The model under review builds one solid part; all positions refer to its coordinate system, in mm. A direction names the side the tool comes from. Coordinates: 2 decimals unless noted, no trailing zeros. Order: outer loops, then holes, each group sorted by start corner. A loop starts at its lowest first (then second) coordinate and runs counter-clockwise, first axis right, second up. Notation, with made-up numbers: (54, 50) -> (68, 50) arc R8 ccw to (68, 62) -> close; hole circle Ø11 at (24.25, 30). An arc over 180 degrees is marked (long way). Put each result on its own line as item: value.
Autodesk Inventor part; units mm, degrees
ref_plane "YZ Plane" through (0, 0, 0) normal (1, 0, 0) x (0, 1, 0)
ref_plane "XZ Plane" through (0, 0, 0) normal (0, 1, 0) x (-1, 0, 0)
ref_plane "XY Plane" through (0, 0, 0) normal (0, 0, 1) x (1, 0, 0)
sketch "Sketch1" plane through (0, 0, 0) normal (0, 0, 1) x (1, 0, 0)
  line L0 (-16.2013, 52.9706) -> (47.2987, 52.9706)
  line L1 (47.2987, 52.9706) -> (47.2987, -10.5294)
  line L2 (47.2987, -10.5294) -> (-16.2013, -10.5294)
  line L3 (-16.2013, -10.5294) -> (-16.2013, 52.9706)
  point P0 (0, 0)
  dimension "d0" = 63.5
  dimension "d1" = 63.5
extrude "Extrusion1" add sketch "Sketch1" along normal blind 6.35
sketch "Sketch2" plane through (0, 0, 6.35) normal (0, 0, 1) x (1, 0, 0)
  line L0 (-16.2013, -10.5294) -> (-16.2013, 52.9706)
  line L1 (47.2987, -10.5294) -> (-16.2013, -10.5294)
  point P0 (0, 0)
  point P1 (15.5487, 21.2206)
  dimension "d4" = 31.75
  dimension "d5" = 31.75
hole "Hole1" at (15.5487, 21.2206, 6.35) direction (0, 0, -1) diameter 44.323 end through all
sketch "Sketch3" plane through (0, 0, 6.35) normal (0, 0, 1) x (1, 0, 0)
  line L0 (47.2987, 52.9706) -> (47.2987, -10.5294)
  line L1 (-16.2013, 52.9706) -> (47.2987, 52.9706)
  line L2 (-16.2013, -10.5294) -> (-16.2013, 52.9706)
  line L3 (47.2987, -10.5294) -> (-16.2013, -10.5294)
  point P0 (0, 0)
  point P1 (-3.5013, 46.6206)
  point P2 (34.5987, 46.6206)
  point P3 (-3.5013, -4.1794)
  point P4 (34.5987, -4.1794)
  dimension "d13" = 6.35
  dimension "d14" = 12.7
  dimension "d15" = 12.7
  dimension "d16" = 6.35
  dimension "d24" = 12.7
  dimension "d25" = 12.7
hole "Hole2" at (-3.5013, 46.6206, 6.35) at (34.5987, 46.6206, 6.35) at (-3.5013, -4.1794, 6.35) at (34.5987, -4.1794, 6.35) direction (0, 0, -1) diameter 6.096 end through all
sketch "Sketch4" plane through (0, 0, 6.35) normal (0, 0, 1) x (1, 0, 0)
  line L0 (-16.2013, 52.9706) -> (47.2987, 52.9706)
  line L1 (-4.7209, 20.4332) -> (-21.033, 20.4332)
  line L2 (-21.033, 20.4332) -> (-21.033, 22.0207)
  line L3 (-21.033, 22.0207) -> (-4.7209, 22.0207)
  line L4 (-4.7209, 22.0207) -> (-4.7209, 20.4332)
  point P0 (0, 0)
  dimension "d26" = 1.5875
  dimension "d27" = 30.9499
extrude "Extrusion2" cut sketch "Sketch4" against normal blind 6.35
sketch "Sketch5" plane through (-16.2013, 52.9706, 0) normal (0, 1, 0) x (1, 0, 0)
  line L0 (0, 0) -> (63.5, 0)
  line L1 (0, 0) -> (0, -6.35)
  point P0 (16.2013, 0)
  point P1 (3.175, -3.175)
  dimension "d30" = 3.175
  dimension "d31" = 3.175
hole "Hole3" at (-13.0263, 52.9706, 3.175) direction (0, -1, 0) diameter 2.6416 depth 50.8 tip angle 118
sketch "Sketch6" plane through (-16.2013, 52.9706, 0) normal (0, 1, 0) x (1, 0, 0)
  circle A0 centre (3.175, -3.175) radius 1.3208
  point P0 (16.2013, 0)
hole "Hole4" at (-13.0263, 52.9706, 3.175) direction (0, -1, 0) diameter 3.81 depth 31.75 tip angle 118
sketch "Sketch7" plane through (0, 0, 0) normal (0, 0, -1) x (-1, 0, 0)
  line L0 (-47.2987, 52.9706) -> (-47.2987, -10.5294)
  line L1 (-40.9487, 22.0207) -> (-35.1672, 22.0207)
  line L2 (-35.1672, 22.0207) -> (-35.1672, 20.4332)
  line L3 (-35.1672, 20.4332) -> (-40.9487, 20.4332)
  line L4 (-40.9487, 20.4332) -> (-40.9487, 22.0207)
  point P0 (0, 0)
  dimension "d46" = 6.35
extrude "Extrusion3" cut sketch "Sketch7" against normal blind 6.35
properties part number "JF-AT-JC0015" material "Aluminum-6061 (Anodized Black)"
Item 1: Consider section D-D on y = 8. Write out the cut boundary in (x, z) (3 decimals), and give its area (3 significant figures).
Answers below:
outline: (-16.201, 0) -> (-2.237, 0) -> (-2.237, 6.35) -> (-16.201, 6.35) -> close; (33.335, 0) -> (47.299, 0) -> (47.299, 6.35) -> (33.335, 6.35) -> close; hole circle Ø2.642 at (-13.026, 3.175)
area: 172 mm^2
Item 2: For faces 1 (the cylindrical face through (-14.336, 11.174, 3.003)), 2 (the flat face through (39, 22.021, 3)), 3 (the flat face through (47.299, 22, 3)), list the 3-axis set-ups (+Z, -Z, +X, -X, +Y, -Y) from which the entire face can be reached by the end or side of a thin tool; tool diameter is ignored.
Answers below:
face 1: +Y
face 2: +Z, -Z, -X
face 3: +Z, -Z, +X, +Y, -Y
Item 3: For line 1 (Y direction, x = -7.5, z = 4); line 2 (X direction, y = 28, z = 4.5); line 3 (X direction, y = 30, z = 3.75), list the stretches that pass through material, from the lowest coordinate up. Write a range as from..to.
Answers below:
line 1: -10.53..20.43, 22.02..52.97
line 2: -16.2..-14.4, -11.66..-5.55, 36.65..47.3
line 3: -16.2..-14.84, -11.21..-4.8, 35.9..47.3
Item 4: Consider section B-B on x = 40. Write out the cut boundary in (y, z).
Answers below:
outline: (-10.53, 0) -> (20.43, 0) -> (20.43, 6.35) -> (-10.53, 6.35) -> close; (22.02, 0) -> (52.97, 0) -> (52.97, 6.35) -> (22.02, 6.35) -> close
Item 5: Consider section C-C on x = -1.5. Write out the cut boundary in (y, z).
Answers below:
outline: (-10.53, 0) -> (-6.48, 0) -> (-6.48, 6.35) -> (-10.53, 6.35) -> close; (-1.88, 0) -> (7.06, 0) -> (7.06, 6.35) -> (-1.88, 6.35) -> close; (35.38, 0) -> (44.32, 0) -> (44.32, 6.35) -> (35.38, 6.35) -> close; (48.92, 0) -> (52.97, 0) -> (52.97, 6.35) -> (48.92, 6.35) -> close
Item 6: Mouldability with a two-part tool opening along Y and no side actions: class faces 4 (the flat face through (8, 43, 6.35)), 5 (the flat face through (16, -10.529, 3)), 6 (the flat face through (-10, 22.021, 3)), 7 (the flat face through (15, 52.971, 3)) as +Y half, -Y half, draft (parallel to the pull), parting line (faces both ways), or undercut.
Answers below:
face 4: draft
face 5: -Y half
face 6: undercut
face 7: +Y half
Item 7: For pin 1 Ø1.9 at (x, z) = (-13, 2.5) entering from +Y; pin 2 Ø5.5 at (x, y) = (34.6, 46.62) entering from -Z; pin 3 Ø2.5 at (x, z) = (-13.03, 3.18) entering from +Y, all flat-tipped, find the tip position at first contact; note any pin that passes through.
Answers below:
pin 1: y = 20.43
pin 2: through
pin 3: y = 2.13
Item 8: Consider section A-A on y = 16. Write out the cut boundary in (x, z) (3 decimals), and give its area (3 significant figures).
Answers below:
outline: (-16.201, 0) -> (-5.989, 0) -> (-5.989, 6.35) -> (-16.201, 6.35) -> close; (37.087, 0) -> (47.299, 0) -> (47.299, 6.35) -> (37.087, 6.35) -> close; hole circle Ø2.642 at (-13.026, 3.175)
area: 124 mm^2
